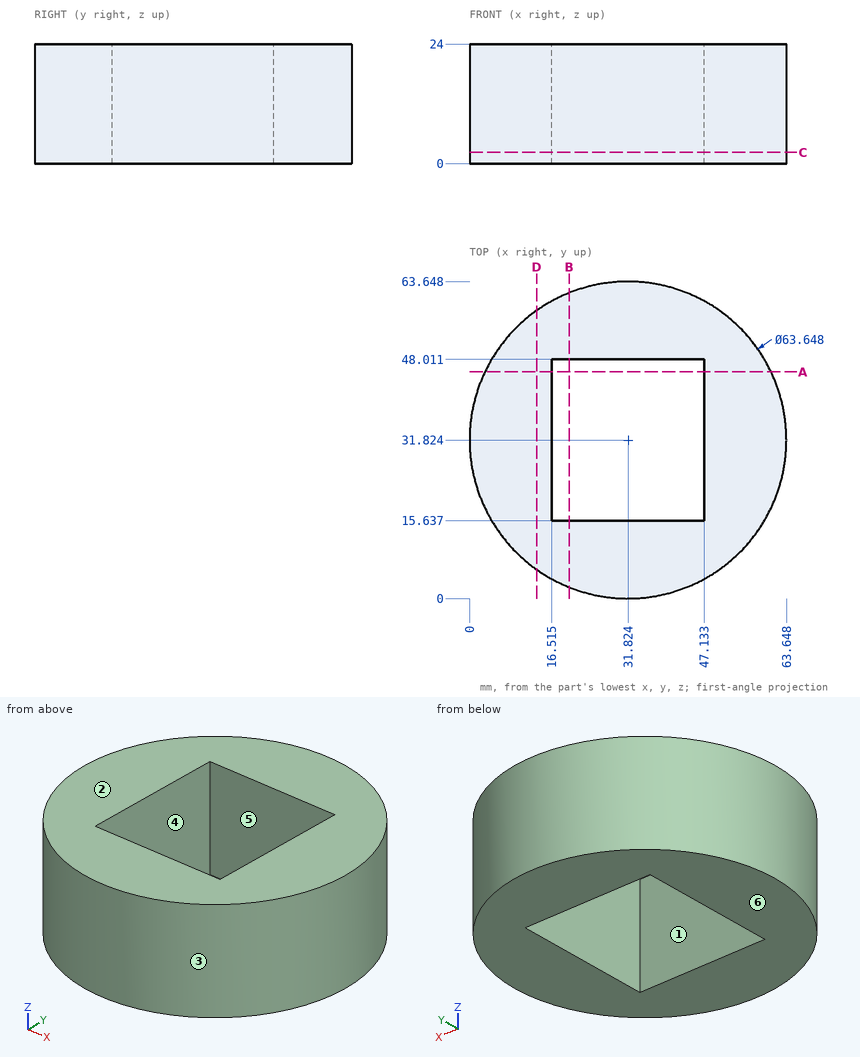
Geometry check sheet. Reference: drawing and pictorial views, mm from the part's lowest x, y, z. A direction names the side the tool comes from. Coordinates: 2 decimals unless noted, no trailing zeros. Loops run counter-clockwise (first coordinate to the right, second up) from the corner with the lowest first, then second, coordinate; pieces in that order, holes last. Notation, with made-up numbers: (39.5, 17.5) -> (81.5, 17.5) arc R16 cw to (81.5, 33.5) -> close; hole circle Ø4 at (61, 12.25). An arc over 180 degrees is marked (long way). Write item = value, one per line. Start each with the question number.
1. Tool access check on the marked faces 5 and 6. Record the directions out of +Z, -Z, +X, -X, +Y, -Y that give a thin tool (end or side, any length) a straight path to the whole face; none if there is none.
2. Draft check along X on the marked faces 1, 2, 3 and 4. Enter one of: released by +X, released by -X, zero draft, split by the parting line, or undercut.
3. Section check B-B on x = 20. Record the cut outline in (y, z), then the cut area to 3 significant figures.
4. Material ranges on line 1 (Y direction, x = 35, z = 20.5); line 2 (X direction, y = 35, z = 9) (1 decimal); line 3 (X direction, y = 29, z = 15.25) (1 decimal), recorded low to high.
5. Section check C-C on z = 2.25. Record the cut outline in (x, y) (1 decimal), then the cut area to 3 significant figures.
6. Depth check by flat-ended pin: P1, Ø8, axis at x = 41.5, z = 6.5, coming from the -Y side; P2, Ø5, axis at x = 24.5, z = 13.5, coming from the +Y side; P3, Ø2, axis at x = 50.5, z = 11, coming from the -Y side. Enter the tip coordinate at first touch or a pass-through.
7. Section check D-D on x = 13.5. Record the cut outline in (y, z) (1 decimal).
8. Section check A-A on y = 45.5. Record the cut outline in (x, z) (1 decimal).
Responses:
q1.face_5 = +Z, -Z
q1.face_6 = -Z, +X, -X, +Y, -Y
q2.face_1 = undercut
q2.face_2 = zero draft
q2.face_3 = split by the parting line
q2.face_4 = undercut
q3.outline = (2.28, 0) -> (15.64, 0) -> (15.64, 24) -> (2.28, 24) -> close; (48.01, 0) -> (61.37, 0) -> (61.37, 24) -> (48.01, 24) -> close
q3.area = 641 mm2
q4.line_1 = 0.16 to 15.64, 48.01 to 63.49
q4.line_2 = 0.2 to 16.5, 47.1 to 63.5
q4.line_3 = 0.1 to 16.5, 47.1 to 63.5
q5.outline = circle Ø63.6 at (31.8, 31.8); hole (16.5, 15.6) -> (47.1, 15.6) -> (47.1, 48) -> (16.5, 48) -> close
q5.area = 2,190 mm2
q6.P1 = 0.51
q6.P2 = 63.28
q6.P3 = 5.36
q7.outline = (5.8, 0) -> (57.8, 0) -> (57.8, 24) -> (5.8, 24) -> close
q8.outline = (3.1, 0) -> (16.5, 0) -> (16.5, 24) -> (3.1, 24) -> close; (47.1, 0) -> (60.6, 0) -> (60.6, 24) -> (47.1, 24) -> close
